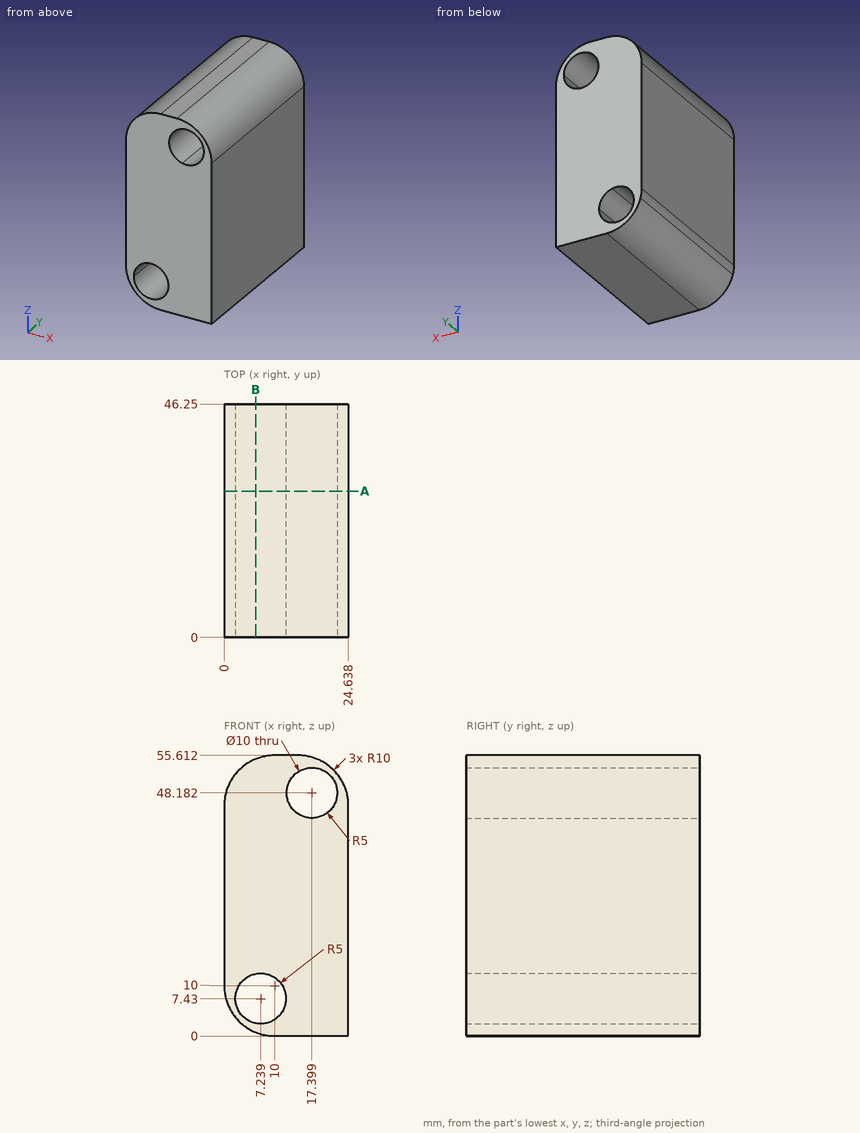
Could you check a few things on this drawing? It's one solid part, dimensions in mm from its lowest x, y, z. Coordinates: 2 decimals unless noted, no trailing zeros. Write each loop counter-clockwise with the first axis right and the second up, starting at its lowest first coordinate (ties: lowest second). Pieces come first, ordered by that corner, then holes.
1) I'm going to push flat-ended pins straight in: pin 1 (10 mm diameter, centred on y = 21, z = 49, fed in from +X); pin 2 (2 mm diameter, centred on y = 26, z = 49, fed in from +X). Where does each tip first touch, or does it pass through?
Filled in:
pin 1: stops at x = 24.64
pin 2: stops at x = 24.35
2) If I drill on line 1 (X direction, y = 42, z = 11); line 2 (Z direction, x = 14.5, y = 22) (1 decimal); line 3 (Z direction, x = 5.75, y = 40.5) (1 decimal), over which ranges is the centre line in solid material (lowest first)?
Filled in:
line 1: x = 0 to 3.74, 10.74 to 24.64
line 2: z = 0 to 44.1, 52.3 to 55.6
line 3: z = 0.9 to 2.7, 12.2 to 54.7
3) If we section it at A-A (y = 29): List the corners of the cut face in (x, z) for me, plus the area to 3 significant figures.
Filled in:
outline: (0, 10) arc R10 ccw to (0.34, 7.43) arc R10 ccw to (10, 0) - (24.64, 0) - (24.64, 45.61) arc R10 ccw to (14.64, 55.61) - (10, 55.61) arc R10 ccw to (0, 45.61) - close; hole (8.45, 12.28) arc R5 ccw (long way) to (12.24, 7.43) arc R5 ccw to start; hole circle Ø10 at (17.4, 48.18)
area: 1,150 mm2
4) If we section it at B-B (x = 6.25): List the corners of the cut face in (y, z) for me.
Filled in:
outline: (0, 0.73) - (46.25, 0.73) - (46.25, 2.53) - (0, 2.53) - close; (0, 12.33) - (46.25, 12.33) - (46.25, 54.88) - (0, 54.88) - close
